```python
from build123d import *

# Parameters (mm, degrees)
SALIENTE_EXTRUIR1_DEPTH    = 55
CROQUIS2_R                 = 9.525
CORTAR_EXTRUIR1_DEPTH      = 3.025
CROQUIS3_W                 = 5.05
CROQUIS3_H                 = 35
CORTAR_EXTRUIR2_DEPTH      = 10
CORTAR_EXTRUIR3_DEPTH      = 79.779756283
CORTAR_EXTRUIR3_DEPTH_BACK = 79.779756283
CROQUIS4_R                 = 5
REDONDEO1_R                = 10
CROQUIS5_R                 = 2.5
CORTAR_EXTRUIR4_DEPTH      = 90.32524839
REDONDEO2_R                = 8


with BuildPart() as part:
    # Croquis1 → Saliente-Extruir1 (new body)
    with BuildSketch(Plane.XY):
        Polygon((-40, 0), (40, 0), (40, -27), (65, -27), (65, -35), (40, -35), (-40, -35), (-65, -35), (-65, -27), (-40, -27), align=None)
    extrude(amount=SALIENTE_EXTRUIR1_DEPTH)

    # Croquis2 → Cortar-Extruir1 (cut, symmetric)
    with BuildSketch(Plane.XY.offset(27.5)):
        Circle(CROQUIS2_R)
    extrude(amount=CORTAR_EXTRUIR1_DEPTH, both=True, mode=Mode.SUBTRACT)

    # Croquis3 → Cortar-Extruir2 (cut)
    with BuildSketch(Plane(origin=(0, 0, 0), x_dir=(1, 0, 0), z_dir=(0, 1, 0))):
        with Locations((-32.475, -27.5)):
            Rectangle(CROQUIS3_W, CROQUIS3_H)
        with Locations((32.475, -27.5)):
            Rectangle(CROQUIS3_W, CROQUIS3_H)
    extrude(amount=-CORTAR_EXTRUIR2_DEPTH, mode=Mode.SUBTRACT)

    # Croquis4 → Cortar-Extruir3 (cut, two sides: drawn at the far end of the back side and taken through both)
    with BuildSketch(Plane.XY.offset(27.5).offset(-CORTAR_EXTRUIR3_DEPTH_BACK)):
        Circle(CROQUIS4_R)
    extrude(amount=CORTAR_EXTRUIR3_DEPTH + CORTAR_EXTRUIR3_DEPTH_BACK, mode=Mode.SUBTRACT)

    # Redondeo1
    redondeo1_edges = [part.edges().sort_by_distance(p)[0] for p in [
        (65, -31, 0),
        (-65, -31, 0),
        (65, -31, 55),
        (-65, -31, 55),
    ]]
    fillet(redondeo1_edges, radius=REDONDEO1_R)

    # Croquis5 → Cortar-Extruir4 (cut, through all)
    with BuildSketch(Plane(origin=(0, -27, 0), x_dir=(1, 0, 0), z_dir=(0, 1, 0))):
        with Locations(Location((-53, -27.5, 0), (0, 0, 270))):
            Circle(CROQUIS5_R)
        with Locations(Location((53, -27.5, 0), (0, 0, 90))):
            Circle(CROQUIS5_R)
    extrude(amount=-CORTAR_EXTRUIR4_DEPTH, mode=Mode.SUBTRACT)

    # Redondeo2
    redondeo2_edges = [part.edges().sort_by_distance(p)[0] for p in [
        (-40, -13.5, 0),
        (40, -13.5, 0),
        (40, -13.5, 55),
        (-40, -13.5, 55),
    ]]
    fillet(redondeo2_edges, radius=REDONDEO2_R)


solid = part.part
```
Design review of the part built by this model. Coordinates are the model's own, in mm. A direction names the side the tool comes from. Coordinates: 2 decimals unless noted, no trailing zeros. Write each loop counter-clockwise with the first axis right and the second up, starting at its lowest first coordinate (ties: lowest second). Pieces come first, ordered by that corner, then holes.
1) Add section A-A (x = -53). Write out the cut boundary in (y, z).
2) Mouldability with a two-part tool opening along Z and no side actions: class faces 1 (the flat face through (32, -10, 27)), 2 (the cylindrical face through (-61.99, -30.94, 52.15)), 3 (the flat face through (-23, 0, 27)) as +Z half, -Z half, draft (parallel to the pull), parting line (faces both ways), or undercut.
3) Machinability: for faces 4 (the cylindrical face through (37.594, -13.689, 2.281)), 5 (the flat face through (32, -5, 10)), 6 (the flat face through (40, -13, 27)), which of the approach directions +Z, -Z, +X, -X, +Y, -Y give a long, thin tool a straight path to every point of the face, cutting with its end or side? Answer none if there is none.
4) Add section D-D (z = 20.5). Write out the cut boundary in (x, y), plus the area to 3 significant figures.
5) Add section B-B (z = 27.5). Write out the cut boundary in (x, y) (3 decimals).
6) Add section C-C (y = -30). Write out the cut boundary in (x, z).
7) To check wall thickness, follow L1, parallel to Z at x = 53, y = -28.5; L2, parallel to X at y = -31.25, z = 27.5; L3, parallel to X at y = -8.5, z = 38.5. State the ranges of each line that lie inside material, in increasing order.
8) Insertion check: pin 1 (2.5 mm diameter, centred on x = -32.5, z = 25.5, fed in from +Y); pin 2 (10.5 mm diameter, centred on x = -0.5, y = -2.5, fed in from +Z); pin 3 (8 mm diameter, centred on y = -5, z = 34.5, fed in from +X); pin 4 (1.5 mm diameter, centred on y = -10, z = 31, fed in from -X). Each pin has a flat end and moves straight along its axis. Give the tip position at first contact, or say it passes through.
Check result:
1. outline: (-35, 0) - (-27, 0) - (-27, 25) - (-35, 25) - close; (-35, 30) - (-27, 30) - (-27, 55) - (-35, 55) - close
2. face 1: undercut
2. face 2: +Z half
2. face 3: draft
3. face 4: -Z, +X, +Y
3. face 5: +Y
3. face 6: +Z, -Z, +X, +Y
4. outline: (-65, -35) - (65, -35) - (65, -27) - (40, -27) - (40, 0) - (35, 0) - (35, -10) - (29.95, -10) - (29.95, 0) - (5, 0) arc R5 cw to (-5, 0) - (-29.95, 0) - (-29.95, -10) - (-35, -10) - (-35, 0) - (-40, 0) - (-40, -27) - (-65, -27) - close
4. area: 3,060 mm2
5. outline: (-65, -35) - (-55.5, -35) - (-55.5, -27) - (-65, -27) - close; (-50.5, -35) - (50.5, -35) - (50.5, -27) - (40, -27) - (40, 0) - (35, 0) - (35, -10) - (29.95, -10) - (29.95, 0) - (9.525, 0) arc R9.525 cw to (-9.525, 0) - (-29.95, 0) - (-29.95, -10) - (-35, -10) - (-35, 0) - (-40, 0) - (-40, -27) - (-50.5, -27) - close; (55.5, -35) - (65, -35) - (65, -27) - (55.5, -27) - close
6. outline: (-65, 10) arc R10 ccw to (-55, 0) - (55, 0) arc R10 ccw to (65, 10) - (65, 45) arc R10 ccw to (55, 55) - (-55, 55) arc R10 ccw to (-65, 45) - close; hole circle Ø5 at (-53, 27.5); hole circle Ø5 at (53, 27.5)
7. L1: z = 0 to 25, 30 to 55
7. L2: x = -65 to -55.5, -50.5 to 50.5, 55.5 to 65
7. L3: x = -40 to -35, -29.95 to 29.95, 35 to 40
8. pin 1: stops at y = -10
8. pin 2: stops at z = 55
8. pin 3: stops at x = 40
8. pin 4: stops at x = -40
